```python
from build123d import *

# Parameters (mm, degrees)
F1_DEPTH = 203.2
F2_R     = 2.54
F3_R     = 2.54


with BuildPart() as f1:
    # F0 (on Front) → F1 (new body, symmetric)
    with BuildSketch(Plane.XZ):
        Polygon((69.85, 12.7), (-69.85, 12.7), (-69.85, -12.7), (-66.675, -12.7), (-66.675, 9.525), (66.675, 9.525), (66.675, -12.7), (69.85, -12.7), align=None)
    extrude(amount=F1_DEPTH, both=True)

    # F2
    f2_edges = [f1.edges().sort_by_distance(p)[0] for p in [
        (-69.85, 0, 12.7),
        (69.85, 0, 12.7),
    ]]
    fillet(f2_edges, radius=F2_R)

    # F3
    f3_edges = [f1.edges().sort_by_distance(p)[0] for p in [
        (-66.675, 0, 9.525),
        (66.675, 0, 9.525),
    ]]
    fillet(f3_edges, radius=F3_R)


solid = f1.part
```
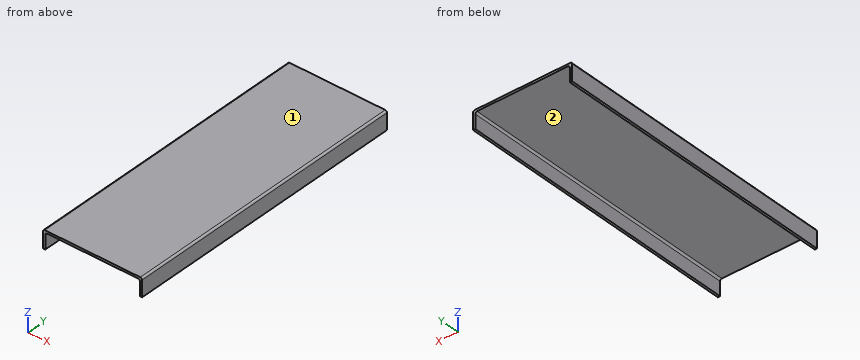
Read the model definition and answer for the solid it produces. Units are mm, in the model's axes. Face numbers are marked on the shaded views. Round coordinates to 2 decimals unless told otherwise and drop trailing zeros. Write each loop counter-clockwise with the first axis right and the second up, starting at its lowest first coordinate (ties: lowest second). Pieces come first, ordered by that corner, then holes. Notation, with made-up numbers: M -7,-17.5 L 3,-17.5 A20 ccw 3,8.5 Z; hole C -38,77 d6. An arc over 180 degrees is marked long. One line per item, written item: value.
Q1. Straight lines are drawn through the part: line 1 (X direction, y = -77, z = 7.5); line 2 (X direction, y = 109, z = 3) (3 decimals); line 3 (Z direction, x = 39, y = -87.5) (3 decimals). For each, find the intervals that lie inside material, in ascending order. Write a range as [from, to].
Data:
line 1: [-69.85, -66.62], [66.62, 69.85]
line 2: [-69.85, -66.675], [66.675, 69.85]
line 3: [9.525, 12.7]
Q2. For a pull along X with two mould halves and no side action, classify the marked faces 1 and 2 as +X half, -X half, draft (parallel to the pull), parting line (faces both ways), or undercut.
Data:
face 1: draft
face 2: undercut
Q3. Find section C-C on x = 39.5. Write down the section's boundary in (y, z) (3 decimals).
Data:
outline: M -203.2,9.525 L 203.2,9.525 L 203.2,12.7 L -203.2,12.7 Z
Q4. Find section B-B on y = 122. Write down the section's boundary in (x, z) (3 decimals), plus the area to 3 significant figures.
Data:
outline: M -69.85,-12.7 L -66.675,-12.7 L -66.675,6.985 A2.54 cw -64.135,9.525 L 64.135,9.525 A2.54 cw 66.675,6.985 L 66.675,-12.7 L 69.85,-12.7 L 69.85,10.16 A2.54 ccw 67.31,12.7 L -67.31,12.7 A2.54 ccw -69.85,10.16 Z
area: 585 mm2
Q5. Find section A-A on z = -6. Write down the section's boundary in (x, y) (3 decimals).
Data:
outline: M -69.85,-203.2 L -66.675,-203.2 L -66.675,203.2 L -69.85,203.2 Z; M 66.675,-203.2 L 69.85,-203.2 L 69.85,203.2 L 66.675,203.2 Z
Q6. A flat-ended cylindrical pin translates along its axis: pin 1 Ø6 at (x, y) = (7, 97.5) entering from -Z (3 decimals). Find the tip coordinate at first contact, or state that the pin passes through.
Data:
pin 1: z = 9.525
